Geometry: final body of the model. Coordinates: model frame, mm. A direction names the side the tool comes from. Coordinates: 2 decimals unless noted, no trailing zeros. Write each loop counter-clockwise with the first axis right and the second up, starting at its lowest first coordinate (ties: lowest second). Pieces come first, ordered by that corner, then holes.
from build123d import *

# Parameters (mm, degrees)
ESQUISSE1_W             = 57
ESQUISSE1_H             = 37
BOSS_EXTRU_1_DEPTH      = 2.5
ESQUISSE2_W             = 7
ESQUISSE2_H             = 15
ENL_V_MAT_EXTRU_1_DEPTH = 69.139562664
ESQUISSE3_W             = 23.5
ESQUISSE3_H             = 10
ENL_V_MAT_EXTRU_2_DEPTH = 69.139562664
ESQUISSE4_W             = 21
ESQUISSE4_H             = 9
ENL_V_MAT_EXTRU_3_DEPTH = 69.139562664
ESQUISSE5_W             = 19
ESQUISSE5_H             = 8
ENL_V_MAT_EXTRU_4_DEPTH = 69.139562664
ESQUISSE6_R             = 2.5
ENL_V_MAT_EXTRU_5_DEPTH = 5
ENL_V_MAT_EXTRU_6_DEPTH = 69.139562664
ESQUISSE8_R             = 1.5
ENL_V_MAT_EXTRU_7_DEPTH = 69.139562664
ESQUISSE9_W             = 25
ESQUISSE9_H             = 1.5
ENL_V_MAT_EXTRU_8_DEPTH = 69.139562664
CONG_1_R                = 5
CONG_2_R                = 1.5
CONG_3_R                = 0.5
CONG_4_R                = 2
CONG_5_R                = 2
TROU_TARAUD_M3_51_D     = 2.9
TROU_TARAUD_M3_51_DEPTH = 12
TROU_TARAUD_M3_51_TIP   = 0.871247898
TROU_TARAUD_M3_52_D     = 2.9
TROU_TARAUD_M3_52_DEPTH = 10
TROU_TARAUD_M3_52_TIP   = 0.871247898
CHANFREIN1_SIZE         = 0.5


with BuildPart() as part:
    # Esquisse1 → Boss.-Extru.1 (new, symmetric)
    with BuildSketch(Plane(origin=(0, 0, 0), x_dir=(0, 0, -1), z_dir=(1, 0, 0))):
        with Locations((-28.5, 18.5)):
            Rectangle(ESQUISSE1_W, ESQUISSE1_H)
    extrude(amount=BOSS_EXTRU_1_DEPTH, both=True)

    # Esquisse2 → Enlèv. mat.-Extru.1 (cut, through all)
    with BuildSketch(Plane(origin=(2.5, 0, 0), x_dir=(0, 0, -1), z_dir=(1, 0, 0))):
        with Locations((-3.5, 14.5)):
            Rectangle(ESQUISSE2_W, ESQUISSE2_H)
    extrude(amount=-ENL_V_MAT_EXTRU_1_DEPTH, mode=Mode.SUBTRACT)

    # Esquisse3 → Enlèv. mat.-Extru.2 (cut, through all)
    with BuildSketch(Plane(origin=(2.5, 0, 0), x_dir=(0, 0, -1), z_dir=(1, 0, 0))):
        with Locations((-18.25, 32)):
            Rectangle(ESQUISSE3_W, ESQUISSE3_H)
    extrude(amount=-ENL_V_MAT_EXTRU_2_DEPTH, mode=Mode.SUBTRACT)

    # Esquisse4 → Enlèv. mat.-Extru.3 (cut, through all)
    with BuildSketch(Plane(origin=(2.5, 0, 0), x_dir=(0, 0, -1), z_dir=(1, 0, 0))):
        with Locations((-46.5, 32.5)):
            Rectangle(ESQUISSE4_W, ESQUISSE4_H)
    extrude(amount=-ENL_V_MAT_EXTRU_3_DEPTH, mode=Mode.SUBTRACT)

    # Esquisse5 → Enlèv. mat.-Extru.4 (cut, through all)
    with BuildSketch(Plane(origin=(2.5, 0, 0), x_dir=(0, 0, -1), z_dir=(1, 0, 0))):
        with Locations((-47.5, 4)):
            Rectangle(ESQUISSE5_W, ESQUISSE5_H)
    extrude(amount=-ENL_V_MAT_EXTRU_4_DEPTH, mode=Mode.SUBTRACT)

    # Esquisse6 → Enlèv. mat.-Extru.5 (cut)
    with BuildSketch(Plane(origin=(2.5, 0, 0), x_dir=(0, 0, -1), z_dir=(1, 0, 0))):
        with BuildLine():
            Line((-57, 28), (-57, 13.5))
            ThreePointArc((-57, 13.5), (-56.994765219, 13.739906631), (-56.97907084, 13.979356585))
            Line((-56.97907084, 13.979356585), (-55.752423485, 28))
            Line((-55.752423485, 28), (-57, 28))
        make_face()
        with BuildLine():
            Line((-57, 8), (-51.5, 8))
            ThreePointArc((-51.5, 8), (-55.389087297, 9.610912703), (-57, 13.5))
            Line((-57, 13.5), (-57, 8))
        make_face()
        with Locations((-51.5, 13.5)):
            Circle(ESQUISSE6_R)
    extrude(amount=-ENL_V_MAT_EXTRU_5_DEPTH, mode=Mode.SUBTRACT)

    # Esquisse7 → Enlèv. mat.-Extru.6 (cut, through all)
    with BuildSketch(Plane(origin=(2.5, 0, 0), x_dir=(0, 0, -1), z_dir=(1, 0, 0))):
        Polygon((-38, 15), (-11, 15), (-11, 4.5), (-30, 4.5), (-30, 10.5), (-38, 10.5), align=None)
    extrude(amount=-ENL_V_MAT_EXTRU_6_DEPTH, mode=Mode.SUBTRACT)

    # Esquisse8 → Enlèv. mat.-Extru.7 (cut, through all)
    with BuildSketch(Plane(origin=(2.5, 0, 0), x_dir=(0, 0, -1), z_dir=(1, 0, 0))):
        with Locations((-19, 19.75)):
            Circle(ESQUISSE8_R)
        with BuildLine():
            Line((-43.75, 22), (-25.25, 22))
            ThreePointArc((-25.25, 22), (-23, 19.75), (-25.25, 17.5))
            Line((-25.25, 17.5), (-43.75, 17.5))
            ThreePointArc((-43.75, 17.5), (-46, 19.75), (-43.75, 22))
        make_face()
    extrude(amount=-ENL_V_MAT_EXTRU_7_DEPTH, mode=Mode.SUBTRACT)

    # Esquisse9 → Enlèv. mat.-Extru.8 (cut, through all)
    with BuildSketch(Plane(origin=(2.5, 0, 0), x_dir=(0, 0, -1), z_dir=(1, 0, 0))):
        with Locations((-18, 0.75)):
            Rectangle(ESQUISSE9_W, ESQUISSE9_H)
    extrude(amount=-ENL_V_MAT_EXTRU_8_DEPTH, mode=Mode.SUBTRACT)

    # Congé1
    # the kernel refuses this fillet: 5 mm, written as the material it adds along each edge
    with BuildSketch(Plane(origin=(2.5, 27, 30), x_dir=(0, 0, -1), z_dir=(-1, 0, 0)), Plane(origin=(2.5, 28, 36), x_dir=(0, 1, 0), z_dir=(-1, 0, 0)), Plane(origin=(2.5, 27, 6.5), x_dir=(0, 1, 0), z_dir=(-1, 0, 0))) as cong_1_piece_1:
        with BuildLine():
            CenterArc((CONG_1_R, -CONG_1_R), CONG_1_R, 90, 90)
            Line((0, -CONG_1_R), (-CONG_1_R * 0.02, -CONG_1_R))
            Line((-CONG_1_R * 0.02, -CONG_1_R), (-CONG_1_R * 0.02, CONG_1_R * 0.02))
            Line((-CONG_1_R * 0.02, CONG_1_R * 0.02), (CONG_1_R, CONG_1_R * 0.02))
            Line((CONG_1_R, CONG_1_R * 0.02), (CONG_1_R, 0))
        make_face()
    extrude(amount=5)
    with BuildSketch(Plane(origin=(2.5, 1.5, 5.5), x_dir=(0, -1, 0), z_dir=(-1, 0, 0))) as cong_1_piece_2:
        with BuildLine():
            CenterArc((5, 3.570714214), CONG_1_R, 180, 45.572995999)
            Line((0, 3.570714214), (-0.1, 3.570714214))
            Line((-0.1, 3.570714214), (-0.1, 0))
            Line((-0.1, 0), (0, -0.1))
            ThreePointArc((0, -0.1), (0.75, -0.1), (1.43, -0.071414284))
            Line((1.43, -0.071414284), (1.5, 0))
        make_face()
    extrude(amount=5)
    with BuildSketch(Plane(origin=(2.5, 1.5, 30.5), x_dir=(0, -1, 0), z_dir=(-1, 0, 0))) as cong_1_piece_3:
        with BuildLine():
            CenterArc((5, -3.570714214), CONG_1_R, 134.427004001, 45.572995999)
            Line((0, -3.570714214), (-0.1, -3.570714214))
            Line((-0.1, -3.570714214), (-0.1, 0))
            Line((-0.1, 0), (0, 0.1))
            ThreePointArc((0, 0.1), (0.75, 0.1), (1.43, 0.071414284))
            Line((1.43, 0.071414284), (1.5, 0))
        make_face()
    extrude(amount=5)

    # Congé2
    cong_2_edges = [part.edges().sort_by_distance(p)[0] for p in [
        (0, 10.5, 38),
        (0, 15, 38),
        (0, 15, 11),
        (0, 4.5, 11),
        (0, 4.5, 30),
    ]]
    fillet(cong_2_edges, radius=CONG_2_R)

    # Congé3
    cong_3_edges = [part.edges().sort_by_distance(p)[0] for p in [
        (0, 10.5, 30),
    ]]
    fillet(cong_3_edges, radius=CONG_3_R)

    # Congé4
    cong_4_edges = [part.edges().sort_by_distance(p)[0] for p in [
        (0, 7, 7),
        (0, 22, 7),
        (0, 8, 38),
    ]]
    fillet(cong_4_edges, radius=CONG_4_R)

    # Congé5
    cong_5_edges = [part.edges().sort_by_distance(p)[0] for p in [
        (0, 28, 55.752423485),
    ]]
    fillet(cong_5_edges, radius=CONG_5_R)

    # Trou taraudé M3.51
    with Locations(Plane(origin=(0, 0, 0), x_dir=(-1, 0, 0), z_dir=(0, -1, 0))):
        with Locations((0, -3), (0, -33)):
            Hole(TROU_TARAUD_M3_51_D / 2, depth=TROU_TARAUD_M3_51_DEPTH)
            with Locations((0, 0, -(TROU_TARAUD_M3_51_DEPTH + TROU_TARAUD_M3_51_TIP / 2))):  # 118° drill point
                Cone(0, TROU_TARAUD_M3_51_D / 2, TROU_TARAUD_M3_51_TIP, mode=Mode.SUBTRACT)

    # Trou taraudé M3.52
    with Locations(Plane(origin=(0, 37, 0), x_dir=(1, 0, 0), z_dir=(0, 1, 0))):
        with Locations((0, -33), (0, -3)):
            Hole(TROU_TARAUD_M3_52_D / 2, depth=TROU_TARAUD_M3_52_DEPTH)
            with Locations((0, 0, -(TROU_TARAUD_M3_52_DEPTH + TROU_TARAUD_M3_52_TIP / 2))):  # 118° drill point
                Cone(0, TROU_TARAUD_M3_52_D / 2, TROU_TARAUD_M3_52_TIP, mode=Mode.SUBTRACT)

    # Chanfrein1
    chanfrein1_edges = [part.edges().sort_by_distance(p)[0] for p in [
        (-2.5, 19.75, 46),
        (-2.5, 22, 34.5),
        (-2.5, 19.75, 23),
        (-2.5, 17.5, 34.5),
        (2.5, 19.75, 46),
        (2.5, 17.5, 34.5),
        (2.5, 19.75, 23),
        (2.5, 22, 34.5),
        (2.5, 1.5, 18),
        (-2.5, 1.5, 18),
        (2.5, 35, 36),
        (-2.5, 35, 36),
        (2.5, 34.5, 6.5),
        (-2.5, 34.5, 6.5),
        (2.5, 27, 18.25),
        (-2.5, 27, 18.25),
        (2.5, 1.109772229, 7.134222541),
        (-2.5, 1.109772229, 7.134222541),
        (2.5, 1.109772229, 28.865777459),
        (-2.5, 1.109772229, 28.865777459),
        (2.5, 29.464466094, 37.464466094),
        (-2.5, 29.464466094, 37.464466094),
        (2.5, 28.464466094, 7.964466094),
        (-2.5, 28.464466094, 7.964466094),
        (2.5, 28.464466094, 28.535533906),
        (-2.5, 28.464466094, 28.535533906),
        (2.5, 15, 24.5),
        (-2.5, 15, 24.5),
        (-2.5, 22, 2.5),
        (2.5, 9.75, 11),
        (-2.5, 9.75, 11),
        (2.5, 4.5, 20.5),
        (-2.5, 4.5, 20.5),
        (2.5, 10.5, 33.5),
        (2.5, 22, 2.5),
        (-2.5, 10.5, 33.5),
        (2.5, 12.75, 38),
        (-2.5, 12.75, 38),
        (2.5, 14.560660172, 11.439339828),
        (-2.5, 14.560660172, 11.439339828),
        (2.5, 4.939339828, 11.439339828),
        (-2.5, 4.939339828, 11.439339828),
        (2.5, 4.939339828, 29.560660172),
        (-2.5, 4.939339828, 29.560660172),
        (2.5, 10.939339828, 37.560660172),
        (-2.5, 10.939339828, 37.560660172),
        (2.5, 14.560660172, 37.560660172),
        (-2.5, 14.560660172, 37.560660172),
        (2.5, 8, 30),
        (-2.5, 8, 30),
        (2.5, 10.353553391, 30.146446609),
        (-2.5, 10.353553391, 30.146446609),
        (2.5, 7, 2.5),
        (-2.5, 7, 2.5),
        (2.5, 14.5, 7),
        (-2.5, 14.5, 7),
        (-2.5, 8, 45.75),
        (2.5, 8, 45.75),
        (2.5, 7.585786438, 6.414213562),
        (-2.5, 7.585786438, 6.414213562),
        (2.5, 21.414213562, 6.414213562),
        (-2.5, 21.414213562, 6.414213562),
        (2.5, 7.414213562, 38.585786438),
        (-2.5, 7.414213562, 38.585786438),
        (2.5, 28, 47.459880569),
        (-2.5, 28, 47.459880569),
        (2.5, 20.076834035, 56.445610687),
        (2.5, 27.474554674, 55.270941553),
        (-2.5, 20.076834035, 56.445610687),
        (-2.5, 27.474554674, 55.270941553),
        (-2.5, 34.5, 30),
        (2.5, 34.5, 30),
        (-2.5, 3, 38),
        (2.5, 3, 38),
        (2.5, 9.784253858, 55.555025352),
        (-2.5, 9.784253858, 55.555025352),
    ]]
    chamfer(chanfrein1_edges, length=CHANFREIN1_SIZE)


solid = part.part
Item 1: Section A-A, the plane z = 19. Output: boundary loops of the cut face in (x, y).
Derived:
outline: (-2.5, 2) - (-2, 1.5) - (2, 1.5) - (2.5, 2) - (2.5, 4) - (2, 4.5) - (-2, 4.5) - (-2.5, 4) - close; (-2.5, 15.5) - (-2, 15) - (2, 15) - (2.5, 15.5) - (2.5, 18.25) - (-2.5, 18.25) - close; (-2.5, 21.25) - (2.5, 21.25) - (2.5, 26.5) - (2, 27) - (-2, 27) - (-2.5, 26.5) - close
Item 2: Material intervals for probe 1 along Y at (x, z) = (-1.5, 25); probe 2 along Y at (x, z) = (0.85, 19); probe 3 along Y at (x, z) = (-0.3, 13.5), sorted ascending.
Derived:
probe 1: y = 1.5 to 4.5, 15 to 17.51, 21.99 to 27
probe 2: y = 1.5 to 4.5, 15 to 18.25, 21.25 to 27
probe 3: y = 1.5 to 4.5, 15 to 27
Item 3: Section B-B, the plane x = 0.7. State how many separate pieces and enclosed holes the cut face has, plus the area to 3 significant figures.
Derived:
separate pieces: 2
enclosed holes: 3
area: 941 mm2
Item 4: Section C-C, the plane y = 24. Output: boundary loops of the cut face in (x, z).
Derived:
outline: (-2.5, 0) - (2.5, 0) - (2.5, 55.6) - (2, 56.1) - (-2, 56.1) - (-2.5, 55.6) - close
Item 5: Set-up query: faces 1 (the conical face through (-2.14, 4.85, 11.33)), 2 (the conical face through (-2.198, 1.215, 6.883)), 3 (the cylindrical face through (-0.03, 10.95, 37.57)), 4 (the cylindrical face through (-0.669, 31.93, 34.286)), 5 (the conical face through (2.135, 14.644, 37.669)). Return all of +Z, -Z, +X, -X, +Y, -Y with unobstructed straight access to the full face (end or side cutting, diameter ignored); none if empty.
Derived:
face 1: -X
face 2: -X, -Y
face 3: +X, -X
face 4: +Y
face 5: +X
Item 6: Pin query (flat end, axial travel): pin 1 (2 mm diameter, centred on x = 1, z = 18.5, fed in from +Y); pin 2 (3 mm diameter, centred on x = -1, z = 38.5, fed in from +Y); pin 3 (1 mm diameter, centred on x = 0, z = 22, fed in from -Y); pin 4 (2.5 mm diameter, centred on y = 19.75, z = 19, fed in from -X). Return the tip coordinate at first contact, or that it passes through.
Derived:
pin 1: stops at y = 27
pin 2: stops at y = 30
pin 3: stops at y = 1.5
pin 4: passes through
Item 7: Pull-direction query (Z, two-part tool) for faces 6 (the conical face through (2.135, 29.329, 37.409)), 7 (the cylindrical face through (-0.03, 4.93, 29.55)), 8 (the flat face through (0, 22, 3)); classes: released by +Z, released by -Z, zero draft, split by the parting line, or undercut.
Derived:
face 6: released by +Z
face 7: undercut
face 8: zero draft
